```python
from build123d import *

# Parameters (mm, degrees)
BOSS_EXTRUDE1_DEPTH = 4.7
SKETCH2_W           = 24.5
SKETCH2_H           = 34.22
SKETCH2_W_2         = 14.75
SKETCH2_H_2         = 15
BOSS_EXTRUDE2_DEPTH = 1.5
SKETCH4_R           = 1.55
BOSS_EXTRUDE3_DEPTH = 3.5
SKETCH5_R           = 1.55
CUT_EXTRUDE1_DEPTH  = 28.197510916
SKETCH6_R           = 2.825
CUT_EXTRUDE2_DEPTH  = 2.5
SKETCH7_R           = 1.55
BOSS_EXTRUDE4_DEPTH = 1.5


with BuildPart() as part:
    # Sketch1 → Boss-Extrude1 (new body)
    with BuildSketch(Plane.XY):
        with BuildLine():
            Line((18.25, -17.11), (15.267630639, 14.179315124))
            ThreePointArc((15.267630639, 14.179315124), (13.331043423, 18.049363172), (9.294701685, 19.61))
            Line((9.294701685, 19.61), (-9.294701685, 19.61))
            ThreePointArc((-9.294701685, 19.61), (-13.331043423, 18.049363172), (-15.267630639, 14.179315124))
            Line((-15.267630639, 14.179315124), (-18.25, -17.11))
            Line((-18.25, -17.11), (-12.25, -17.11))
            Line((-12.25, -17.11), (-12.25, 17.11))
            Line((-12.25, 17.11), (12.25, 17.11))
            Line((12.25, 17.11), (12.25, -17.11))
            Line((12.25, -17.11), (18.25, -17.11))
        make_face()
    extrude(amount=BOSS_EXTRUDE1_DEPTH)

    # Sketch2 → Boss-Extrude2 (add)
    # profile 1 of 2: a face of its own
    with BuildSketch(Plane.XY.offset(4.7)):
        Rectangle(SKETCH2_W, SKETCH2_H)
        with Locations((0, -0.11)):
            Rectangle(SKETCH2_W_2, SKETCH2_H_2, mode=Mode.SUBTRACT)
    # profile 2 of 2: a face of its own
    with BuildSketch(Plane.XY.offset(4.7)):
        with BuildLine():
            Line((12.25, 17.11), (12.25, -17.11))
            Line((12.25, -17.11), (18.25, -17.11))
            Line((18.25, -17.11), (15.267630639, 14.179315124))
            ThreePointArc((15.267630639, 14.179315124), (13.331043423, 18.049363172), (9.294701685, 19.61))
            Line((9.294701685, 19.61), (-9.294701685, 19.61))
            ThreePointArc((-9.294701685, 19.61), (-13.331043423, 18.049363172), (-15.267630639, 14.179315124))
            Line((-15.267630639, 14.179315124), (-18.25, -17.11))
            Line((-18.25, -17.11), (-12.25, -17.11))
            Line((-12.25, -17.11), (-12.25, 17.11))
            Line((-12.25, 17.11), (12.25, 17.11))
        make_face()
    extrude(amount=BOSS_EXTRUDE2_DEPTH)

    # Sketch4 → Boss-Extrude3 (add)
    with BuildSketch(Plane(origin=(0, 0, 4.7), x_dir=(-1, 0, 0), z_dir=(0, 0, -1))):
        with BuildLine():
            Line((-12.25, 17.11), (-7.25, 17.11))
            Line((-7.25, 17.11), (-7.25, 13.51))
            ThreePointArc((-7.25, 13.51), (-7.689339828, 12.449339828), (-8.75, 12.01))
            Line((-8.75, 12.01), (-12.25, 12.01))
            Line((-12.25, 12.01), (-12.25, 17.11))
        make_face()
        with Locations((-10.2, 14.86)):
            Circle(SKETCH4_R, mode=Mode.SUBTRACT)
    boss_extrude3 = extrude(amount=BOSS_EXTRUDE3_DEPTH)

    # Sketch5 → Cut-Extrude1 (cut, through all)
    with BuildSketch(Plane(origin=(0, 0, 4.7), x_dir=(-1, 0, 0), z_dir=(0, 0, -1))):
        with Locations((-10.2, 14.86)):
            Circle(SKETCH5_R)
    extrude(amount=-CUT_EXTRUDE1_DEPTH, mode=Mode.SUBTRACT)

    # Sketch6 → Cut-Extrude2 (cut)
    with BuildSketch(Plane.XY.offset(6.2)):
        with Locations((10.2, 14.86)):
            Circle(SKETCH6_R)
    cut_extrude2 = extrude(amount=-CUT_EXTRUDE2_DEPTH, mode=Mode.SUBTRACT)

    # Sketch7 → Boss-Extrude4 (add)
    with BuildSketch(Plane.XZ.offset(17.11)):
        with BuildLine():
            Line((-22.25, 6.2), (-18.25, 6.2))
            ThreePointArc((-18.25, 6.2), (-15.15, 3.1), (-18.25, 0))
            Line((-18.25, 0), (-22.25, 0))
            ThreePointArc((-22.25, 0), (-25.35, 3.1), (-22.25, 6.2))
        make_face()
        with Locations(Location((-22.25, 3.1, 0), (0, 0, 270))):
            Circle(SKETCH7_R, mode=Mode.SUBTRACT)
    boss_extrude4 = extrude(amount=-BOSS_EXTRUDE4_DEPTH)

    # Mirror1: Boss-Extrude3, Cut-Extrude2, Boss-Extrude4 across plane
    add(boss_extrude3.mirror(Plane(origin=(0, 0, 0), x_dir=(0, 0, 1), z_dir=(1, 0, 0))))
    add(cut_extrude2.mirror(Plane(origin=(0, 0, 0), x_dir=(0, 0, 1), z_dir=(1, 0, 0))), mode=Mode.SUBTRACT)
    add(boss_extrude4.mirror(Plane(origin=(0, 0, 0), x_dir=(0, 0, 1), z_dir=(1, 0, 0))))


solid = part.part
```
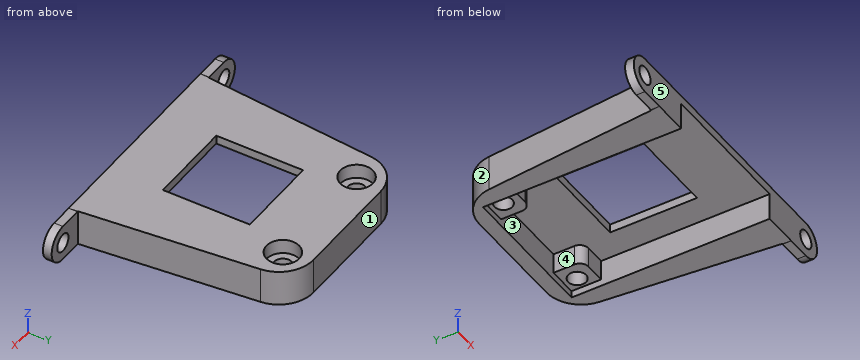
Check sheet for the modelled part. Datum: model origin and axes. Units: mm. Face numbers are marked on the shaded views. A direction names the side the tool comes from. Coordinates: 2 decimals unless noted, no trailing zeros. Write each loop counter-clockwise with the first axis right and the second up, starting at its lowest first coordinate (ties: lowest second). Pieces come first, ordered by that corner, then holes. Notation, with made-up numbers: M 47.5,-8.5 L 106.5,-8.5 A10 cw 106.5,8.5 Z; hole C 48,68.25 d5. An arc over 180 degrees is marked long. Use one line per item in the form item = value.
Item 1: Material ranges on L1, parallel to Y at x = 1.5, z = 5.5; L2, parallel to Z at x = -7, y = 12.5; L3, parallel to Z at x = 22.25, y = -16.4, recorded low to high. Write a range as from..to.
Answer below:
L1 = -17.11..-7.61, 7.39..19.61
L2 = 4.7..6.2
L3 = 0..1.55, 4.65..6.2
Item 2: Sectioned sample at A-A, the plane z = 3.1. State how many separate pieces and enclosed holes the cut face has, and give its area (3 significant figures).
Answer below:
separate_pieces = 3
enclosed_holes = 2
area = 408 mm^2
Item 3: Sectioned sample at C-C, the plane y = 14.86. Record the cut outline in (x, z) (3 decimals).
Answer below:
outline = M -15.163,0 L -12.25,0 L -12.25,1.2 L -11.75,1.2 L -11.75,3.7 L -13.025,3.7 L -13.025,6.2 L -15.163,6.2 Z; M -8.65,1.2 L -7.25,1.2 L -7.25,4.7 L 7.25,4.7 L 7.25,1.2 L 8.65,1.2 L 8.65,3.7 L 7.375,3.7 L 7.375,6.2 L -7.375,6.2 L -7.375,3.7 L -8.65,3.7 Z; M 11.75,1.2 L 12.25,1.2 L 12.25,0 L 15.163,0 L 15.163,6.2 L 13.025,6.2 L 13.025,3.7 L 11.75,3.7 Z
Item 4: Sectioned sample at D-D, the plane y = -2. Record the cut outline in (x, z) (3 decimals), and give its area (3 significant figures).
Answer below:
outline = M -16.81,0 L -12.25,0 L -12.25,4.7 L -7.375,4.7 L -7.375,6.2 L -16.81,6.2 Z; M 7.375,4.7 L 12.25,4.7 L 12.25,0 L 16.81,0 L 16.81,6.2 L 7.375,6.2 Z
area = 71.2 mm^2
Item 5: Gauge pin test, flat ends, axial feed: pin 1 Ø3 at (x, z) = (-6, 1.5) entering from -Y; pin 2 Ø3 at (x, z) = (20, 3) entering from +Y; pin 3 Ø1 at (x, y) = (14.5, 9) entering from -Z; pin 4 Ø4.5 at (x, y) = (10.2, 14.86) entering from +Z. Record the tip position at first contact, or that the pin passes through.
Answer below:
pin_1 = 12.68
pin_2 = -15.61
pin_3 = 0
pin_4 = 3.7
Item 6: Set-up check for the marked faces 4 and 5: record each of +Z, -Z, +X, -X, +Y, -Y from which the full face is reachable in a straight line by a thin tool's end or side.
Answer below:
face_4 = -Z, -Y
face_5 = +Z, -Z, +X, -X, -Y
Item 7: Release check for a two-part mould opening along X. For the marked faces 1, 2 and 3 record: pulls with the +X half, pulls with the -X half, needs draft (parallel to the pull), parting line crosses it, or undercut.
Answer below:
face_1 = needs draft
face_2 = pulls with the -X half
face_3 = undercut
Item 8: Sectioned sample at B-B, the plane x = -6. Record the cut outline in (y, z).
Answer below:
outline = M -17.11,4.7 L -7.61,4.7 L -7.61,6.2 L -17.11,6.2 Z; M 7.39,4.7 L 17.11,4.7 L 17.11,0 L 19.61,0 L 19.61,6.2 L 7.39,6.2 Z
